Work out the finished part from the listing and answer in its coordinate system (mm). Face numbers are marked on the shaded views. A direction names the side the tool comes from. Give positions to 0.01 mm unless a question says otherwise; leave off trailing zeros. Loops run counter-clockwise (first coordinate to the right, second up) from the corner with the lowest first, then second, coordinate; pieces in that order, holes last. Notation, with made-up numbers: (-10.5, 55) - (-6.5, 55) arc R19 cw to (-6.5, 80) - close; hole circle Ø1 at (74.5, 67). An arc over 180 degrees is marked (long way). One line per question, with ' | ' between items. Start each with the question number.
1. Find the intervals of material crossed by line 1 (Y direction, x = 14.25, z = 0.75); line 2 (Y direction, x = 0, z = 0.65); line 3 (Z direction, x = -2.5, y = 14.5), in increasing order.
2. Which of the six approach directions +Z, -Z, +X, -X, +Y, -Y give full straight-line access (tool end or side, diameter ignored) to the marked faces 3 and 4?
3. Section A-A (z = 0.55) is taken. Determine the outline of the cut face in (x, y), plus the area to 3 significant figures.
4. Section B-B (y = 12) is taken. Give the number of separate pieces and of enclosed holes in the cut face, plus the area to 3 significant figures.
5. Each of these flat-tipped pins is pushed along its axis until it touches: pin 1 (11 mm diameter, centred on x = -1.5, y = -1, fed in from +Z); pin 2 (5 mm diameter, centred on x = -14.25, y = -12, fed in from -Z); pin 3 (3.5 mm diameter, centred on x = 14.25, y = 12, fed in from -Z). Where does it stop, or does it pass through?
6. For a pull along Y with two mould halves and no side action, classify the marked faces 1 and 2 as released by +Y, released by -Y, zero draft, split by the parting line, or undercut.
from build123d import *

# Parameters (mm, degrees)
SKETCH_2_R          = 2
EXTRUDE_1_DEPTH     = 1
FILLET_1_R          = 10
FILLET_2_R          = 10
SKETCH_4_R          = 4
CUT_EXTRUDE_1_DEPTH = 10
SKETCH_5_R          = 7
CUT_EXTRUDE_2_DEPTH = 1


with BuildPart() as part:
    # 草图2 → 凸台-拉伸1 (new body)
    with BuildSketch(Plane.XY):
        with BuildLine():
            Line((-14.25, 15), (14.25, 15))
            ThreePointArc((14.25, 15), (16.785462764, 13.603567451), (16.960523709, 10.714285714))
            ThreePointArc((16.960523709, 10.714285714), (14.548221281, 0), (16.960523709, -10.714285714))
            ThreePointArc((16.960523709, -10.714285714), (16.785462764, -13.603567451), (14.25, -15))
            Line((14.25, -15), (-14.25, -15))
            ThreePointArc((-14.25, -15), (-16.785462764, -13.603567451), (-16.960523709, -10.714285714))
            ThreePointArc((-16.960523709, -10.714285714), (-14.548221281, 0), (-16.960523709, 10.714285714))
            ThreePointArc((-16.960523709, 10.714285714), (-16.785462764, 13.603567451), (-14.25, 15))
        make_face()
        with Locations((14.25, 12)):
            Circle(SKETCH_2_R, mode=Mode.SUBTRACT)
        with Locations((-14.25, 12)):
            Circle(SKETCH_2_R, mode=Mode.SUBTRACT)
        with Locations((-14.25, -12)):
            Circle(SKETCH_2_R, mode=Mode.SUBTRACT)
        with Locations((14.25, -12)):
            Circle(SKETCH_2_R, mode=Mode.SUBTRACT)
    extrude(amount=EXTRUDE_1_DEPTH)

    # 草图3 → 旋转1 (revolve)
    with BuildSketch(Plane(origin=(0, 0, 0), x_dir=(1, 0, 0), z_dir=(0, 1, 0)), mode=Mode.PRIVATE) as revolve_1_sk:
        Polygon((0, 1), (8, 1), (12, 0), (0, 0), align=None)
    revolve(revolve_1_sk.sketch.rotate(Axis((0, 0, 0), (0, 0, 1)), 180), axis=Axis((0, 0, 0), (0, 0, 1)))

    # 圆角1
    fillet_1_edges = [part.edges().sort_by_distance(p)[0] for p in [
        (12, 0, 0),
    ]]
    fillet(fillet_1_edges, radius=FILLET_1_R)

    # 圆角2
    fillet_2_edges = [part.edges().sort_by_distance(p)[0] for p in [
        (8, 0, -1),
    ]]
    fillet(fillet_2_edges, radius=FILLET_2_R)

    # 草图4 → 切除-拉伸1 (cut)
    with BuildSketch(Plane(origin=(0, 0, -1), x_dir=(-1, 0, 0), z_dir=(0, 0, -1))):
        Circle(SKETCH_4_R)
    extrude(amount=-CUT_EXTRUDE_1_DEPTH, mode=Mode.SUBTRACT)

    # 草图5 → 切除-拉伸2 (cut)
    with BuildSketch(Plane.XY.offset(1)):
        Circle(SKETCH_5_R)
    extrude(amount=-CUT_EXTRUDE_2_DEPTH, mode=Mode.SUBTRACT)


solid = part.part
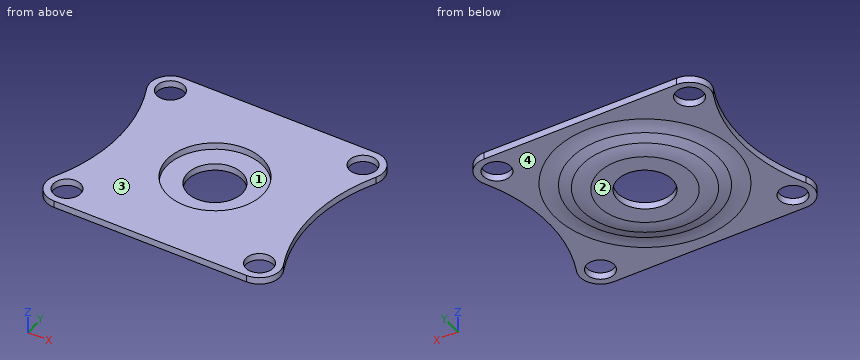
Conclusion:
1) line 1: -15 to -14, -10 to 10, 14 to 15 | line 2: -15 to -7, 7 to 15 | line 3: 0 to 1
2) face 3: +Z, +X, -X, +Y, -Y | face 4: -Z
3) outline: (-16.96, -10.71) arc R3 ccw to (-14.25, -15) - (14.25, -15) arc R3 ccw to (16.96, -10.71) arc R25 cw to (16.96, 10.71) arc R3 ccw to (14.25, 15) - (-14.25, 15) arc R3 ccw to (-16.96, 10.71) arc R25 cw to start; hole circle Ø4 at (-14.25, -12); hole circle Ø4 at (-14.25, 12); hole circle Ø14 at (0, 0); hole circle Ø4 at (14.25, -12); hole circle Ø4 at (14.25, 12) | area: 741 mm²
4) separate pieces: 3 | enclosed holes: 0 | area: 26.9 mm²
5) pin 1: z = 1 | pin 2: z = 0 | pin 3: through
6) face 1: undercut | face 2: zero draft
